```python
from build123d import *

# Parameters (mm, degrees)
ESQUISSE1_R             = 13
BOSS_EXTRU_1_DEPTH      = 12
BOSS_EXTRU_2_START      = -12
ESQUISSE2_R             = 13
ESQUISSE2_R_2           = 5.5
BOSS_EXTRU_2_DEPTH      = 3
ESQUISSE4_R             = 8
ENL_V_MAT_EXTRU_2_DEPTH = 6
ESQUISSE5_R             = 3
ENL_V_MAT_EXTRU_3_DEPTH = 69.271516755
ENL_V_START             = -12
ESQUISSE6_W             = 10
ESQUISSE6_H             = 6
ENL_V_MAT_EXTRU_4_DEPTH = 12
CHANFREIN1_SIZE         = 5
ESQUISSE7_R             = 1
ENL_V_MAT_EXTRU_5_DEPTH = 12
ESQUISSE8_W             = 80
ESQUISSE8_H             = 9
ENL_V_MAT_EXTRU_6_DEPTH = 70.057946682


with BuildPart() as part:
    # Esquisse1 → Boss.-Extru.1 (new body)
    with BuildSketch(Plane.XY):
        Polygon((-40, 0), (40, 0), (40, 25), (17, 25), (17, 55), (-17, 55), (-17, 25), (-40, 25), align=None)
        with Locations((0, 40)):
            Circle(ESQUISSE1_R, mode=Mode.SUBTRACT)
    extrude(amount=BOSS_EXTRU_1_DEPTH)

    # Esquisse2 → Boss.-Extru.2 (add)
    with BuildSketch(Plane.XY.offset(12).offset(BOSS_EXTRU_2_START)):
        with Locations((0, 40)):
            Circle(ESQUISSE2_R)
        with Locations((0, 40)):
            Circle(ESQUISSE2_R_2, mode=Mode.SUBTRACT)
    extrude(amount=BOSS_EXTRU_2_DEPTH)

    # Esquisse4 → Enlèv. mat.-Extru.2 (cut)
    with BuildSketch(Plane(origin=(0, 0, 0), x_dir=(-1, 0, 0), z_dir=(0, 0, -1))):
        with Locations((-25, 15)):
            Circle(ESQUISSE4_R)
        with Locations(Location((25, 15, 0), (0, 0, 180))):
            Circle(ESQUISSE4_R)
    extrude(amount=-ENL_V_MAT_EXTRU_2_DEPTH, mode=Mode.SUBTRACT)

    # Esquisse5 → Enlèv. mat.-Extru.3 (cut, through all)
    with BuildSketch(Plane(origin=(0, 0, 6), x_dir=(-1, 0, 0), z_dir=(0, 0, -1))):
        with Locations((-25, 15)):
            Circle(ESQUISSE5_R)
        with Locations(Location((25, 15, 0), (0, 0, 180))):
            Circle(ESQUISSE5_R)
    extrude(amount=-ENL_V_MAT_EXTRU_3_DEPTH, mode=Mode.SUBTRACT)

    # Esquisse6 → Enlèv. mat.-Extru.4 (cut)
    with BuildSketch(Plane.XY.offset(12).offset(ENL_V_START)):
        with Locations((35, 3)):
            Rectangle(ESQUISSE6_W, ESQUISSE6_H)
        with Locations((-35, 3)):
            Rectangle(ESQUISSE6_W, ESQUISSE6_H)
    extrude(amount=ENL_V_MAT_EXTRU_4_DEPTH, mode=Mode.SUBTRACT)

    # Chanfrein1
    chanfrein1_edges = [part.edges().sort_by_distance(p)[0] for p in [
        (-17, 55, 6),
        (17, 55, 6),
        (17, 25, 6),
        (40, 25, 6),
        (-40, 25, 6),
        (-17, 25, 6),
    ]]
    chamfer(chanfrein1_edges, length=CHANFREIN1_SIZE)

    # Esquisse7 → Enlèv. mat.-Extru.5 (cut)
    with BuildSketch(Plane(origin=(0, 0, 0), x_dir=(-1, 0, 0), z_dir=(0, 0, -1))):
        with Locations((-10, 45)):
            Circle(ESQUISSE7_R)
        with Locations(Location((10, 45, 0), (0, 0, 180))):
            Circle(ESQUISSE7_R)
        with Locations((-37, 15)):
            Circle(ESQUISSE7_R)
        with Locations(Location((37, 15, 0), (0, 0, 180))):
            Circle(ESQUISSE7_R)
        with Locations((0, 15)):
            Circle(ESQUISSE7_R)
    extrude(amount=-ENL_V_MAT_EXTRU_5_DEPTH, mode=Mode.SUBTRACT)

    # Esquisse8 → Enlèv. mat.-Extru.6 (cut, through all)
    with BuildSketch(Plane(origin=(0, 55, 0), x_dir=(1, 0, 0), z_dir=(0, 1, 0))):
        with Locations((0, -4.5)):
            Rectangle(ESQUISSE8_W, ESQUISSE8_H)
    extrude(amount=-ENL_V_MAT_EXTRU_6_DEPTH, mode=Mode.SUBTRACT)


solid = part.part
```
Design review of the part built by this model. Coordinates are the model's own, in mm. A direction names the side the tool comes from. Round coordinates to 2 decimals unless told otherwise and drop trailing zeros. Write each loop counter-clockwise with the first axis right and the second up, starting at its lowest first coordinate (ties: lowest second). Pieces come first, ordered by that corner, then holes. Notation, with made-up numbers: (14, 66.25) -> (46, 66.25) arc R26 cw to (46, 102.25) -> close; hole circle Ø4 at (1.5, 26). An arc over 180 degrees is marked (long way). Answer in a Markdown table with one row per item.
Q1. For faces 1 (the face through (-17, 40, 10)), 2 (the face through (35, 6, 10)), 3 (the face through (29, 25, 10)), list the 3-axis set-ups (+Z, -Z, +X, -X, +Y, -Y) from which the entire face can be reached by the end or side of a thin tool; tool diameter is ignored.
The answers:
| item | result |
|---|---|
| face 1 | +Z, -Z, -X, +Y |
| face 2 | +Z, -Z, +X, -Y |
| face 3 | +Z, -Z, +X, +Y |
Q2. To check wall thickness, follow L1, parallel to Y at x = 0, z = 9.8; L2, parallel to X at y = 40, z = 11.05; L3, parallel to Y at x = 25, z = 9.85. State the ranges of each line that lie inside material, in increasing order. Write a range as [from, to].
The answers:
| item | result |
|---|---|
| L1 | [0, 14], [16, 27], [53, 55] |
| L2 | [-17, -13], [13, 17] |
| L3 | [0, 12], [18, 25] |
Q3. Clearance check with flat-ended pins moving along their axes: pin 1 Ø0.9 at (x, z) = (-31.5, 11) entering from +Y; pin 2 Ø1 at (y, z) = (23.5, 11.5) entering from -X; pin 3 Ø1.5 at (y, z) = (4, 11) entering from +X. State where each tip first meets the part, or that it passes through.
The answers:
| item | result |
|---|---|
| pin 1 | y = 25 |
| pin 2 | x = -37 |
| pin 3 | x = 30 |
Q4. Take a section at C-C, the plane x = 0. State the section outline as (y, z) points, then the cut area to 3 significant figures.
The answers:
| item | result |
|---|---|
| outline | (0, 9) -> (14, 9) -> (14, 12) -> (0, 12) -> close; (16, 9) -> (27, 9) -> (27, 12) -> (16, 12) -> close; (53, 9) -> (55, 9) -> (55, 12) -> (53, 12) -> close |
| area | 81.0 mm² |
Q5. Take a section at D-D, the plane y = 48. State the section outline as (x, z) points.
The answers:
| item | result |
|---|---|
| outline | (-17, 9) -> (-10.25, 9) -> (-10.25, 12) -> (-17, 12) -> close; (10.25, 9) -> (17, 9) -> (17, 12) -> (10.25, 12) -> close |
Q6. Take a section at B-B, the plane z = 11.35. State the section outline as (x, y) points, then the cut area to 3 significant figures.
The answers:
| item | result |
|---|---|
| outline | (-40, 6) -> (-30, 6) -> (-30, 0) -> (30, 0) -> (30, 6) -> (40, 6) -> (40, 20) -> (35, 25) -> (22, 25) -> (17, 30) -> (17, 50) -> (12, 55) -> (-12, 55) -> (-17, 50) -> (-17, 30) -> (-22, 25) -> (-35, 25) -> (-40, 20) -> close; hole circle Ø2 at (-37, 15); hole circle Ø6 at (-25, 15); hole circle Ø26 at (0, 40); hole circle Ø2 at (0, 15); hole circle Ø6 at (25, 15); hole circle Ø2 at (37, 15) |
| area | 2,280 mm² |
Q7. Draft analysis for pull direction X (two halves, no side actions). For faces 4 (the face through (-37, 23, 10)), 5 (the face through (38, 22, 10)), 6 (the face through (-35, 6, 10)), 7 (the face through (-1.69, 52.89, 10.48)), state which applies: +X half, -X half, draft (parallel to the pull), parting line (faces both ways), or undercut.
The answers:
| item | result |
|---|---|
| face 4 | -X half |
| face 5 | +X half |
| face 6 | draft |
| face 7 | undercut |
Q8. Take a section at A-A, the plane x = -37. State the section outline as (y, z) points, then the cut area to 3 significant figures.
The answers:
| item | result |
|---|---|
| outline | (6, 9) -> (14, 9) -> (14, 12) -> (6, 12) -> close; (16, 9) -> (23, 9) -> (23, 12) -> (16, 12) -> close |
| area | 45.0 mm² |
